Geometry check sheet. Reference: drawing and pictorial views, mm from the part's lowest x, y, z. A direction names the side the tool comes from. Give positions to 0.01 mm unless a question says otherwise; leave off trailing zeros. Write each loop counter-clockwise with the first axis right and the second up, starting at its lowest first coordinate (ties: lowest second). Pieces come first, ordered by that corner, then holes. Notation, with made-up numbers: (49, -9.75) -> (68, -9.75) arc R31 ccw to (68, 24.25) -> close; hole circle Ø10 at (-5, 36). An arc over 180 degrees is marked (long way). Write each question's results on one line, items separated by ' | '. Start each with the question number.
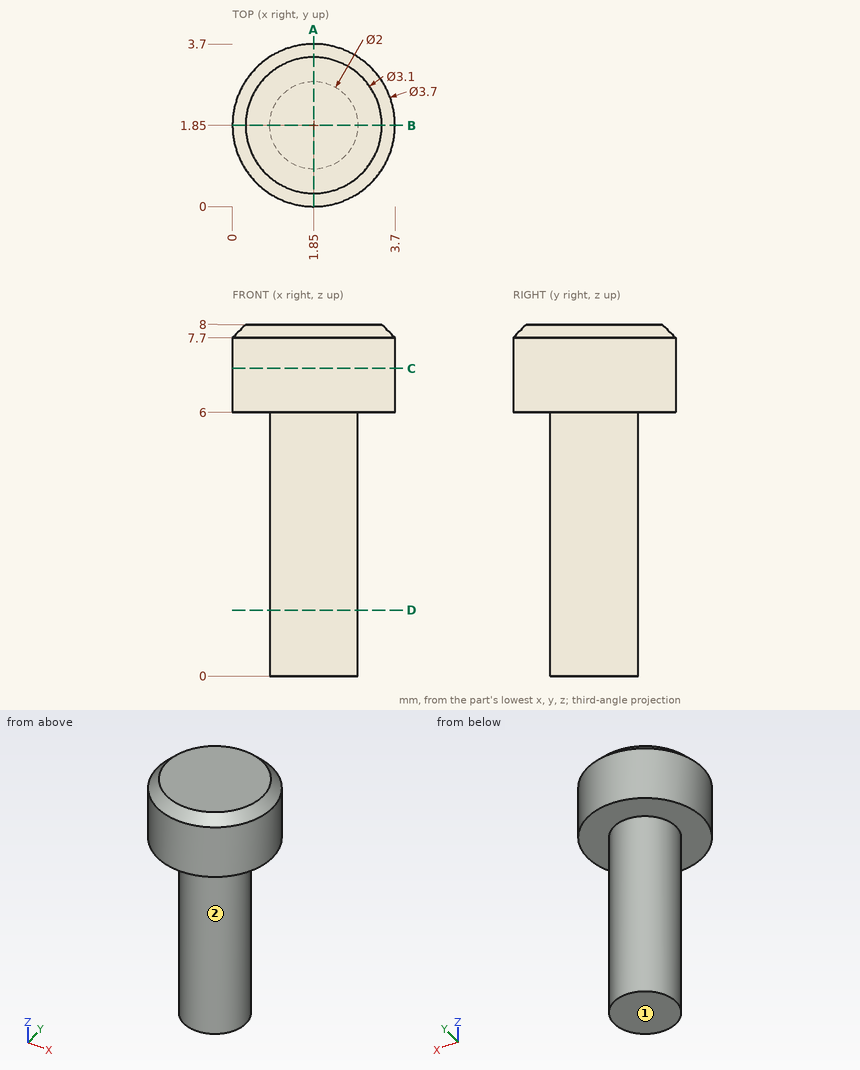
Item 1: Section check C-C on z = 7. Record the boundary of the cut face in (x, y), then the cut area to 3 significant figures.
Item 2: Section check D-D on z = 1.5. Record the boundary of the cut face in (x, y).
Item 3: Thickness scan on probe 1 along Z at (x, y) = (1, 2.75); probe 2 along Y at (x, z) = (1.05, 1); probe 3 along Z at (x, y) = (3.25, 0.8). Record the ranges inside material, lowest first. Write a range as from..to.
Item 4: Section check A-A on x = 1.85. Record the boundary of the cut face in (y, z).
Item 5: Depth check by flat-ended pin: pin 1 Ø1.5 at (x, z) = (2, 1) entering from -Y; pin 2 Ø2 at (x, z) = (0.5, 7) entering from -Y. Enter the tip coordinate at first touch or a pass-through.
Item 6: Set-up check for the marked faces 1 and 2: record each of +Z, -Z, +X, -X, +Y, -Y from which the full face is reachable in a straight line by a thin tool's end or side.
Check sheet entries:
1) outline: circle Ø3.7 at (1.85, 1.85) | area: 10.8 mm^2
2) outline: circle Ø2 at (1.85, 1.85)
3) probe 1: z = 6..8 | probe 2: y = 1.25..2.45 | probe 3: z = 6..7.8
4) outline: (0, 6) -> (0.85, 6) -> (0.85, 0) -> (2.85, 0) -> (2.85, 6) -> (3.7, 6) -> (3.7, 7.7) -> (3.4, 8) -> (0.3, 8) -> (0, 7.7) -> close
5) pin 1: stops at y = 0.85 | pin 2: stops at y = 0.03
6) face 1: -Z, +X, -X, +Y, -Y | face 2: -Z
